from build123d import *

# Parameters (mm, degrees)
SKETCH2_R          = 1.752085735
CUT_EXTRUDE2_DEPTH = 4
CHAMFER1_SIZE      = 1


with BuildPart() as part:
    # Sketch1 → Revolve1 (revolve)
    with BuildSketch(Plane.XY):
        Polygon((-55, 1), (-55, 0), (-62.5, 0), (-62.5, 4), (-41, 4), (-41, 1), align=None)
    revolve(axis=Axis((0, 0, 0), (0, 1, 0)))

    # Sketch2 → Cut-Extrude2 (cut, through all)
    with BuildSketch(Plane.XZ.offset(-1)):
        with Locations((-48, 0)):
            Circle(SKETCH2_R)
        with Locations((-14.83281573, 45.650712782)):
            Circle(SKETCH2_R)
        with Locations((38.83281573, 28.21369211)):
            Circle(SKETCH2_R)
        with Locations((38.83281573, -28.21369211)):
            Circle(SKETCH2_R)
        with Locations((-14.83281573, -45.650712782)):
            Circle(SKETCH2_R)
    extrude(amount=-CUT_EXTRUDE2_DEPTH, mode=Mode.SUBTRACT)

    # Chamfer1
    chamfer1_edges = [part.edges().sort_by_distance(p)[0] for p in [
        (62.5, 4, 0),
        (41, 4, 0),
    ]]
    chamfer(chamfer1_edges, length=CHAMFER1_SIZE)


solid = part.part
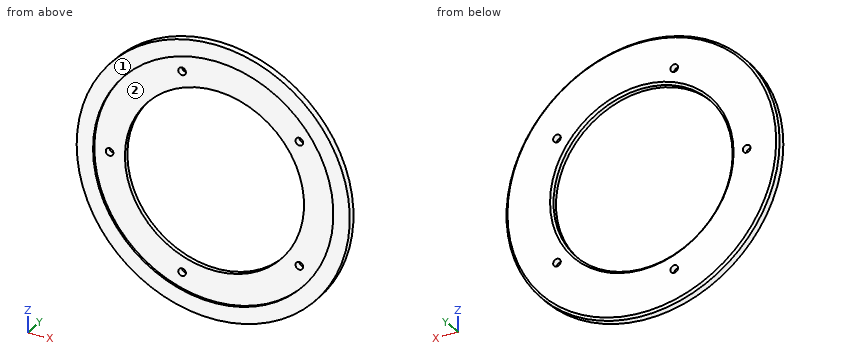
Model file for the job. Use its own axes, mm. Face numbers are marked on the shaded views. Round coordinates to 2 decimals unless told otherwise and drop trailing zeros. Loops run counter-clockwise (first coordinate to the right, second up) from the corner with the lowest first, then second, coordinate; pieces in that order, holes last. Notation, with made-up numbers: (-21, 71.5) -> (36, 71.5) arc R15 ccw to (36, 96.5) -> close; hole circle Ø1 at (-8, 86.25). An arc over 180 degrees is marked (long way). Answer as CSV lines item,"result". Start each with the question number.
1) Slice it at B-B (z = 0). List the corners of the cut face in (x, y), plus the area to 3 significant figures.
2) Slice it at A-A (x = 0). List the corners of the cut face in (y, z).
3) Slice it at C-C (y = 1.95). List the corners of the cut face in (x, z).
4) Mould opens along Z. For the marked faces 1 and 2 say: +Z half, -Z half, draft (parallel to the pull), parting line (faces both ways), or undercut.
5) Pin check, flat tips, straight feed: P1, Ø4.5, axis at x = 38.83, z = -28.21, coming from the -Y side; P2, Ø1.5, axis at y = 2.5, z = -7, coming from the +X side. Stop position of each tip, or through.
6) Probe line 1 along Y through (x, z) = (-36, -28.5); line 2 along X through (y, z) = (0.5, -38.5); line 3 along Z through (x, y) = (24.5, 1.3). List the from-to ranges inside material, lowest first.
Filled in:
1,outline,"(-62.5, 0) -> (-55, 0) -> (-55, 1) -> (-49.75, 1) -> (-49.75, 4) -> (-61.5, 4) -> (-62.5, 3) -> close; (-46.25, 1) -> (-41, 1) -> (-41, 3) -> (-42, 4) -> (-46.25, 4) -> close; (41, 1) -> (55, 1) -> (55, 0) -> (62.5, 0) -> (62.5, 3) -> (61.5, 4) -> (42, 4) -> (41, 3) -> close"
1,area,"131 mm2"
2,outline,"(0, -62.5) -> (3, -62.5) -> (4, -61.5) -> (4, -42) -> (3, -41) -> (1, -41) -> (1, -55) -> (0, -55) -> close; (0, 55) -> (1, 55) -> (1, 41) -> (3, 41) -> (4, 42) -> (4, 61.5) -> (3, 62.5) -> (0, 62.5) -> close"
3,outline,"circle Ø125 at (0, 0); hole circle Ø3.5 at (-48, 0); hole circle Ø82 at (0, 0); hole circle Ø3.5 at (-14.83, -45.65); hole circle Ø3.5 at (-14.83, 45.65); hole circle Ø3.5 at (38.83, -28.21); hole circle Ø3.5 at (38.83, 28.21)"
4,face 1,"draft"
4,face 2,"undercut"
5,P1,"stops at y = 1"
5,P2,"stops at x = 62.19"
6,line 1,"y = 1 to 4"
6,line 2,"x = -49.23 to -39.28, 39.28 to 49.23"
6,line 3,"z = -57.5 to -32.87, 32.87 to 57.5"
